Here's how the part is built. I have some questions about the finished solid (model axes, mm). A direction names the side the tool comes from. Round coordinates to 2 decimals unless told otherwise and drop trailing zeros. Write each loop counter-clockwise with the first axis right and the second up, starting at its lowest first coordinate (ties: lowest second). Pieces come first, ordered by that corner, then holes. Notation, with made-up numbers: (30.25, 77) - (50.25, 77) arc R14 ccw to (50.25, 100) - close; hole circle Ø4 at (-23.75, 3.5). An arc over 180 degrees is marked (long way). One line per question, with ' | ' between items. Start each with the question number.
(1) If I drill on L1, parallel to Y at x = -0.75, z = -7.75; L2, parallel to Z at x = 0, y = -2.75; L3, parallel to Y at x = -1, z = -11, over which ranges is the centre line in solid material (lowest first)?
(2) Imagine slicing it at A-A (x = 0). Write out the boundary of the cut face in (y, z).
(3) For faces 4 (the flat face through (0, -1, 0)), 5 (the flat face through (0, 5, 0)), which set-ups out of +Z, -Z, +X, -X, +Y, -Y let a thin tool reach every point of the face, with its end or its side?
(4) Imagine slicing it at C-C (y = 2.75). Write out the boundary of the cut face in (x, z).
(5) Will these pins go through, and if not, where does the flat tip stop? pin 1 (3 mm diameter, centred on y = 1, z = -4.5, fed in from +X); pin 2 (1.5 mm diameter, centred on y = 0, z = 7, fed in from +X); pin 3 (1 mm diameter, centred on x = -2, z = -5.5, fed in from -Y).
(6) Imagine slicing it at B-B (y = -2.5). Write out the boundary of the cut face in (x, z).
(7) Thinking about a two-plate mould opening in Z: for faces 1 (the cylindrical face through (-1.405, -2.521, 10.703)), 2 (the flat face through (-9, 0, -6)), 3 (the cylindrical face through (10.158, 2.465, 3.199)), which applies, pulls with the +Z half, pulls with the -Z half, needs draft (parallel to the pull), parting line crosses it, or undercut?
from build123d import *

# Parameters (mm, degrees)
F0_R     = 10.65
F1_DEPTH = 5
F0_R_2   = 11.9
F2_DEPTH = 4
F2_TAPER = 10
F3_R     = 10.7946920772
F4_DEPTH = 3


with BuildPart() as f1:
    # F0 (on Front) → F1 (new body)
    with BuildSketch(Plane.XZ):
        Circle(F0_R)
    extrude(amount=-F1_DEPTH)

    # F0 (on Front) → F2 (join)
    with BuildSketch(Plane.XZ):
        Circle(F0_R_2)
        Circle(F0_R, mode=Mode.SUBTRACT)
        Circle(F0_R)
    extrude(amount=F2_DEPTH, taper=F2_TAPER)

    # F3 (on face) → F4 (cut)
    with BuildSketch(Plane.XZ.offset(4)):
        Circle(F3_R)
    extrude(amount=-F4_DEPTH, mode=Mode.SUBTRACT)


solid = f1.part
Check sheet entries:
1) L1: -1 to 5 | L2: -11.42 to -10.79, 10.79 to 11.42 | L3: -4 to 0
2) outline: (-4, -11.19) - (0, -11.9) - (0, -10.65) - (5, -10.65) - (5, 10.65) - (0, 10.65) - (0, 11.9) - (-4, 11.19) - (-4, 10.79) - (-1, 10.79) - (-1, -10.79) - (-4, -10.79) - close
3) face 4: -Y | face 5: +Z, -Z, +X, -X, +Y
4) outline: circle Ø21.3 at (0, 0)
5) pin 1: x = 11.41 | pin 2: x = 10.13 | pin 3: y = -1
6) outline: circle Ø22.92 at (0, 0); hole circle Ø21.59 at (0, 0)
7) face 1: undercut | face 2: needs draft | face 3: parting line crosses it
